Print and shaded views of the part. All mm, measured from the part's lowest x, y and z. A direction names the side the tool comes from. Round coordinates to 2 decimals unless told otherwise and drop trailing zeros. Order: outer loops, then holes, each group sorted by start corner. A loop starts at its lowest first (then second) coordinate and runs counter-clockwise, first axis right, second up. Notation, with made-up numbers: (16, 42) - (64, 42) arc R25 cw to (64, 62) - close; hole circle Ø3 at (-22.5, 89). An arc over 180 degrees is marked (long way). Write item = value, one per line. Start each with the question number.
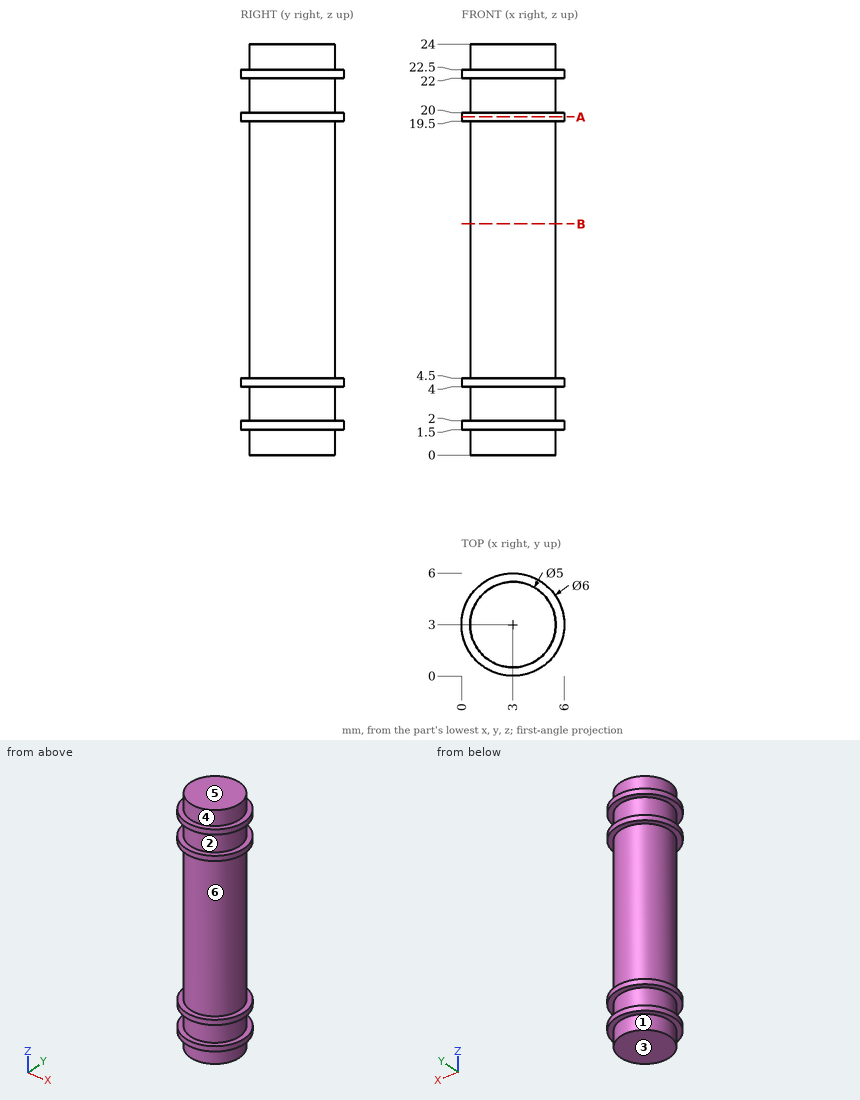
Item 1: Mould opens along Z. For the marked faces 3, 4, 5 and 6 say: +Z half, -Z half, draft (parallel to the pull), parting line (faces both ways), or undercut.
Item 2: Drop flat-ended pins along their axis: pin 1 (1 mm diameter, centred on y = 3.5, z = 15, fed in from +X); pin 2 (1.5 mm diameter, centred on x = 5, z = 13.5, fed in from +Y); pin 3 (3 mm diameter, centred on x = 4, z = 11, fed in from +Y). Give the stop position or say it passes through.
Item 3: Saw through at B-B, the plane z = 13.5. Give the cut face in (x, y).
Item 4: Probe L1, parallel to Z at x = 2.55, y = 5.7; L2, parallel to Y at x = 3.05, z = 12.5. List the from-to ranges inside material, lowest first.
Item 5: Which spindle directions (+Z, -Z, +X, -X, +Y, -Y) get a long thin tool onto all of the face, cutting with end or side? Do the marked faces 1 and 2. Say none if no direction does.
Item 6: Saw through at A-A, the plane z = 19.75. Give the cut face in (x, y).
Check sheet entries:
q1.face_3 = -Z half
q1.face_4 = draft
q1.face_5 = +Z half
q1.face_6 = undercut
q2.pin_1 = 5.5
q2.pin_2 = 5.17
q2.pin_3 = 5.5
q3.outline = circle Ø5 at (3, 3)
q4.L1 = 1.5 to 2, 4 to 4.5, 19.5 to 20, 22 to 22.5
q4.L2 = 0.5 to 5.5
q5.face_1 = -Z
q5.face_2 = none
q6.outline = circle Ø6 at (3, 3)
